from build123d import *

# Parameters (mm, degrees)
F0_W        = 20.1
F0_H        = 22.7
F0_W_2      = 18.5
F0_H_2      = 21.1
F1_DEPTH    = 14
F2_DEPTH    = 1
F3_W        = 0.8
F3_H        = 12
F4_DEPTH    = 11
F5_W        = 0.8
F5_H        = 2
F6_DEPTH    = 1
F7_W        = 0.8
F7_H        = 2
F8_DEPTH    = 1
F9_T4_DEPTH = 11.0867319519
F9_T9_DEPTH = 11.0867319519


# Not quite as in the source:
# - a fillet or chamfer that OpenCascade refuses, or shapes differently, is made with other operations: its cross-section is extruded or revolved along the edge and cut away or added


with BuildPart() as f1:
    # F0 (on Top) → F1 (new body)
    with BuildSketch(Plane.XY):
        Rectangle(F0_W, F0_H)
        Rectangle(F0_W_2, F0_H_2, mode=Mode.SUBTRACT)
    extrude(amount=F1_DEPTH)

    # F0 (on Top) → F2 (join)
    with BuildSketch(Plane.XY):
        Rectangle(F0_W_2, F0_H_2)
    extrude(amount=F2_DEPTH)

    # F3 (on face) → F4 (cut)
    with BuildSketch(Plane.XY.offset(14)):
        with Locations((9.65, 0)):
            Rectangle(F3_W, F3_H)
    extrude(amount=-F4_DEPTH, mode=Mode.SUBTRACT)

    # F5 (on face) → F6 (join)
    with BuildSketch(Plane.XZ.offset(-6)):
        with Locations((9.65, 6.45)):
            Rectangle(F5_W, F5_H)
    extrude(amount=F6_DEPTH)

    # F7 (on face) → F8 (join)
    with BuildSketch(Plane(origin=(0, -6, 0), x_dir=(-1, 0, 0), z_dir=(0, 1, 0))):
        with Locations((-9.65, 6.45)):
            Rectangle(F7_W, F7_H)
    extrude(amount=F8_DEPTH)

    # F9: chamfer of 2 on 2 edges, made by hand


with BuildPart() as f9_tool2:
    # F9_s3 → F9_t4 (new body)
    with BuildSketch(Plane.YZ.offset(15.1933659759)):
        Polygon((5, 5.45), (7, 7.45), (5, 7.45), align=None)
    extrude(amount=-F9_T4_DEPTH)

    split(bisect_by=Plane.XZ.offset(-6), keep=Keep.TOP)


with BuildPart() as f1_1:
    add(f1.part)

    # F9_t1: cut F9_tool2
    add(f9_tool2.part, mode=Mode.SUBTRACT)


with BuildPart() as f9_tool7:
    # F9_s8 → F9_t9 (new body)
    with BuildSketch(Plane.YZ.offset(4.1066340241)):
        Polygon((-7, 7.45), (-5, 5.45), (-5, 7.45), align=None)
    extrude(amount=F9_T9_DEPTH)

    split(bisect_by=Plane.XZ.offset(6), keep=Keep.BOTTOM)


with BuildPart() as f1_2:
    add(f1_1.part)

    # F9_t6: cut F9_tool7
    add(f9_tool7.part, mode=Mode.SUBTRACT)


solid = f1_2.part
Source: CAD feature listing. Evaluate the final solid. Frame: model axes, mm. A direction names the side the tool comes from. Round coordinates to 2 decimals unless told otherwise and drop trailing zeros. Loops run counter-clockwise (first coordinate to the right, second up) from the corner with the lowest first, then second, coordinate; pieces in that order, holes last. Notation, with made-up numbers: (4, 73.25) - (9, 73.25) arc R18 cw to (9, 103.25) - close; hole circle Ø5 at (57.5, 68.5). An arc over 180 degrees is marked (long way). Write item = value, one per line. Start each with the question number.
(1) Pin query (flat end, axial travel): pin 1 (5.5 mm diameter, centred on x = 0.5, y = -1, fed in from +Z). Return the tip coordinate at first contact, or that it passes through.
(2) Section query D-D, the plane x = 3.25. Output: boundary loops of the cut face in (y, z).
(3) Pull-direction query (Y, two-part tool) for faces 3 (the face through (10.05, 0, 2)), 4 (the face through (0, -10.55, 7)), 5 (the face through (0, 11.35, 7)); classes: +Y half, -Y half, draft (parallel to the pull), parting line (faces both ways), or undercut.
(4) Section query B-B, the plane y = -5.5. Output: boundary loops of the cut face in (x, z).
(5) Section query A-A, the plane z = 2. Output: boundary loops of the cut face in (x, y).
(6) Set-up query: faces 1 (the face through (-9.25, 0, 7)), 2 (the face through (9.7, -5.5, 5.45)). Return all of +Z, -Z, +X, -X, +Y, -Y with unobstructed straight access to the full face (end or side cutting, diameter ignored); none if empty.
(7) Ray query, line 1 along X through (y, z) = (6.5, 10.75); line 2 along Y through (x, z) = (1, 4); line 3 along X through (y, z) = (1.75, 8.5). Return the intervals inside material, ascending. Write a range as from..to.
(8) Section query C-C, the plane z = 5.75. Output: boundary loops of the cut face in (x, y).
Conclusion:
q1.pin_1 = 1
q2.outline = (-11.35, 0) - (11.35, 0) - (11.35, 14) - (10.55, 14) - (10.55, 1) - (-10.55, 1) - (-10.55, 14) - (-11.35, 14) - close
q3.face_3 = draft
q3.face_4 = undercut
q3.face_5 = +Y half
q4.outline = (-10.05, 0) - (10.05, 0) - (10.05, 3) - (9.25, 3) - (9.25, 1) - (-9.25, 1) - (-9.25, 14) - (-10.05, 14) - close; (9.25, 5.45) - (10.05, 5.45) - (10.05, 5.95) - (9.25, 5.95) - close
q5.outline = (-10.05, -11.35) - (10.05, -11.35) - (10.05, 11.35) - (-10.05, 11.35) - close; hole (-9.25, -10.55) - (9.25, -10.55) - (9.25, 10.55) - (-9.25, 10.55) - close
q6.face_1 = +Z
q6.face_2 = +X
q7.line_1 = -10.05..-9.25, 9.25..10.05
q7.line_2 = -11.35..-10.55, 10.55..11.35
q7.line_3 = -10.05..-9.25
q8.outline = (-10.05, -11.35) - (10.05, -11.35) - (10.05, -5.3) - (9.25, -5.3) - (9.25, -10.55) - (-9.25, -10.55) - (-9.25, 10.55) - (9.25, 10.55) - (9.25, 5.3) - (10.05, 5.3) - (10.05, 11.35) - (-10.05, 11.35) - close
